from build123d import *

# Parameters (mm, degrees)
SKETCH2_R                        = 21.59
SKETCH2_R_2                      = 10.922
BOSS_EXTRUDE1_DEPTH              = 38.1
CUT_EXTRUDE1_REACH               = 50.825
SKETCH3_W                        = 21.59
SKETCH3_H                        = 1.5875
CUT_EXTRUDE2_REACH               = 50.825
SKETCH4_R                        = 3.0226
TAP_DRILL_FOR_M4X0_7_TAP1_REACH  = 54.717
TAP_DRILL_FOR_M4X0_7_TAP1_BORE_R = 1.65
CUT_EXTRUDE5_REACH               = 63.5
CUT_EXTRUDE5_END_RADIUS          = 3.0226
SKETCH11_R                       = 1.65
CUT_EXTRUDE6_REACH               = 50.825
TAP_DRILL_FOR_M3X0_5_TAP2_D      = 2.5
TAP_DRILL_FOR_M3X0_5_TAP2_DEPTH  = 4.572
TAP_DRILL_FOR_M3X0_5_TAP2_TIP    = 0.751075774


with BuildPart() as part:
    # Sketch2 → Boss-Extrude1 (new body)
    with BuildSketch(Plane(origin=(0, 0, 0), x_dir=(1, 0, 0), z_dir=(0, 1, 0))):
        with Locations(Location((0, 0, 0), (0, 0, 90))):
            Circle(SKETCH2_R)
        with Locations(Location((0, 0, 0), (0, 0, 90))):
            Circle(SKETCH2_R_2, mode=Mode.SUBTRACT)
    extrude(amount=BOSS_EXTRUDE1_DEPTH)

    # Sketch3 → Cut-Extrude1 (cut, up to next)
    with BuildSketch(Plane(origin=(0, 38.1, 0), x_dir=(1, 0, 0), z_dir=(0, 1, 0)), mode=Mode.PRIVATE) as cut_extrude1_sk1:
        with Locations((-10.795, 0)):
            Rectangle(SKETCH3_W, SKETCH3_H)
    cut_extrude1_tool1 = extrude(cut_extrude1_sk1.sketch, amount=-CUT_EXTRUDE1_REACH, mode=Mode.PRIVATE) & part.part
    add(cut_extrude1_tool1.solids().sort_by_distance((-10.795, 38.1, 0))[0], mode=Mode.SUBTRACT)

    # Sketch4 → Cut-Extrude2 (cut, up to next)
    with BuildSketch(Plane(origin=(0, 38.1, 0), x_dir=(1, 0, 0), z_dir=(0, 1, 0)), mode=Mode.PRIVATE) as cut_extrude2_sk1:
        with Locations(Location((0, -16.256, 0), (0, 0, 270))):
            Circle(SKETCH4_R)
    cut_extrude2_tool1 = extrude(cut_extrude2_sk1.sketch, amount=-CUT_EXTRUDE2_REACH, mode=Mode.PRIVATE) & part.part
    cut_extrude2 = cut_extrude2_tool1.solids().sort_by_distance((0, 38.1, 16.256))[0]
    add(cut_extrude2, mode=Mode.SUBTRACT)

    # Tap Drill for M4x0.7 Tap1 bore (on position points) → Tap Drill for M4x0.7 Tap1 (cut, up to next)
    with BuildSketch(Plane(origin=(-16.234261615, 29.109235595, 0.79375), x_dir=(-1, 0, 0), z_dir=(0, 0, -1)), mode=Mode.PRIVATE) as tap_drill_for_m4x0_7_tap1_sk1:
        Circle(TAP_DRILL_FOR_M4X0_7_TAP1_BORE_R)
    tap_drill_for_m4x0_7_tap1_tool1 = extrude(tap_drill_for_m4x0_7_tap1_sk1.sketch, amount=-TAP_DRILL_FOR_M4X0_7_TAP1_REACH, mode=Mode.PRIVATE) & part.part
    # Tap Drill for M4x0.7 Tap1 bore (on position points) → Tap Drill for M4x0.7 Tap1 (cut, up to next)
    with BuildSketch(Plane(origin=(-16.234261615, 29.109235595, 0.79375), x_dir=(-1, 0, 0), z_dir=(0, 0, -1)), mode=Mode.PRIVATE) as tap_drill_for_m4x0_7_tap1_sk2:
        with Locations((0, -20.205281104)):
            Circle(TAP_DRILL_FOR_M4X0_7_TAP1_BORE_R)
    tap_drill_for_m4x0_7_tap1_tool2 = extrude(tap_drill_for_m4x0_7_tap1_sk2.sketch, amount=-TAP_DRILL_FOR_M4X0_7_TAP1_REACH, mode=Mode.PRIVATE) & part.part
    add(tap_drill_for_m4x0_7_tap1_tool1.solids().sort_by_distance((-16.234262, 29.109236, 0.79375))[0], mode=Mode.SUBTRACT)
    add(tap_drill_for_m4x0_7_tap1_tool2.solids().sort_by_distance((-16.234262, 8.903954, 0.79375))[0], mode=Mode.SUBTRACT)

    # Cut-Extrude5: up to this cylinder (the profile starts outside it)
    cut_extrude5_end = Plane(origin=(0, 19.05, 16.256), z_dir=(0, 1, 0)) * Cylinder(CUT_EXTRUDE5_END_RADIUS, 134.0452, mode=Mode.PRIVATE)
    # Sketch11 → Cut-Extrude5 (cut, up to the surface)
    with BuildSketch(Plane.XY.offset(21.59), mode=Mode.PRIVATE) as cut_extrude5_sk1:
        with Locations((0.007297963, 19.05)):
            Circle(SKETCH11_R)
    cut_extrude5_tool1 = extrude(cut_extrude5_sk1.sketch, amount=-CUT_EXTRUDE5_REACH, mode=Mode.PRIVATE) - cut_extrude5_end
    cut_extrude5 = cut_extrude5_tool1.solids().sort_by_distance((0.007298, 19.05, 21.59))[0]
    add(cut_extrude5, mode=Mode.SUBTRACT)

    # Mirror1: Cut-Extrude2, Cut-Extrude5 across plane
    add(cut_extrude2.mirror(Plane.XY), mode=Mode.SUBTRACT)
    add(cut_extrude5.mirror(Plane.XY), mode=Mode.SUBTRACT)

    # Sketch12 → Cut-Extrude6 (cut, up to next)
    with BuildSketch(Plane(origin=(0, 38.1, 0), x_dir=(1, 0, 0), z_dir=(0, 1, 0)), mode=Mode.PRIVATE) as cut_extrude6_sk1:
        with BuildLine():
            Line((20.32, 7.295594561), (20.32, -7.295594561))
            ThreePointArc((20.32, -7.295594561), (21.59, 0), (20.32, 7.295594561))
        make_face()
    cut_extrude6_tool1 = extrude(cut_extrude6_sk1.sketch, amount=-CUT_EXTRUDE6_REACH, mode=Mode.PRIVATE) & part.part
    add(cut_extrude6_tool1.solids().sort_by_distance((20.829303, 38.1, 0))[0], mode=Mode.SUBTRACT)

    # Tap Drill for M3x0.5 Tap2
    with Locations(Plane(origin=(20.32, 19.05, 0), x_dir=(0, 0, 1), z_dir=(1, 0, 0))):
        with Locations((0, 0)):
            Hole(TAP_DRILL_FOR_M3X0_5_TAP2_D / 2, depth=TAP_DRILL_FOR_M3X0_5_TAP2_DEPTH)
            with Locations((0, 0, -(TAP_DRILL_FOR_M3X0_5_TAP2_DEPTH + TAP_DRILL_FOR_M3X0_5_TAP2_TIP / 2))):  # 118° drill point
                Cone(0, TAP_DRILL_FOR_M3X0_5_TAP2_D / 2, TAP_DRILL_FOR_M3X0_5_TAP2_TIP, mode=Mode.SUBTRACT)


solid = part.part
Source: CAD feature listing. Evaluate the final solid. Frame: model axes, mm. A direction names the side the tool comes from. Give positions to 0.01 mm unless a question says otherwise; leave off trailing zeros. Order: outer loops, then holes, each group sorted by start corner. A loop starts at its lowest first (then second) coordinate and runs counter-clockwise, first axis right, second up. Notation, with made-up numbers: (-11.5, 70) -> (19.5, 70) arc R19 cw to (19.5, 87) -> close; hole circle Ø10 at (56, 49.25). An arc over 180 degrees is marked (long way). Write item = value, one per line.
Item 1: Set-up query: faces 4 (the face through (-16, 19, 0.794)), 5 (the face through (0.769, 17.586, 20.207)), 6 (the face through (0.769, 17.586, -20.207)). Return all of +Z, -Z, +X, -X, +Y, -Y with unobstructed straight access to the full face (end or side cutting, diameter ignored); none if empty.
Check result:
face_4 = -X, +Y, -Y
face_5 = +Z
face_6 = -Z
Item 2: Section query C-C (x = -13). Output: boundary loops of the cut face in (y, z).
Check result:
outline = (0, -17.24) -> (38.1, -17.24) -> (38.1, -0.79) -> (0, -0.79) -> close; (0, 0.79) -> (38.1, 0.79) -> (38.1, 17.24) -> (0, 17.24) -> close
Item 3: Section query D-D (z = -12). Output: boundary loops of the cut face in (x, y), then the cut area to 3 significant figures.
Check result:
outline = (-17.95, 0) -> (17.95, 0) -> (17.95, 38.1) -> (-17.95, 38.1) -> close
area = 1,370 mm²
Item 4: Contact query for flat-ended pins moving along their axis: pin 1 (1.5 mm diameter, centred on y = 19.05, z = 0, fed in from +X); pin 2 (4.5 mm diameter, centred on x = -16.23, y = 29.11, fed in from +Z); pin 3 (3 mm diameter, centred on x = -15, y = 22, fed in from -Z); pin 4 (4.5 mm diameter, centred on x = 0.01, y = 19.05, fed in from +Z). Output: stop coordinate, or through.
Check result:
pin_1 = 15.45
pin_2 = 16.45
pin_3 = -16.85
pin_4 = 21.59
Item 5: Section query A-A (y = 24). Output: boundary loops of the cut face in (x, z), then the cut area to 3 significant figures.
Check result:
outline = (-21.58, -0.79) arc R21.59 ccw to (20.32, -7.3) -> (20.32, 7.3) arc R21.59 ccw to (-21.58, 0.79) -> (-10.89, 0.79) arc R10.92 cw (long way) to (-10.89, -0.79) -> close; hole circle Ø6.05 at (0, -16.26); hole circle Ø6.05 at (0, 16.26)
area = 1,000 mm²
Item 6: Mould query, pull axis Z, two halves, no side actions, for faces 1 (the face through (18.002, 17.996, -0.672)), 2 (the face through (-3.723, 18.783, 21.267)), 3 (the face through (-14.586, 29.182, 8.251)). Classes: +Z half, -Z half, draft (parallel to the pull), parting line (faces both ways), or undercut.
Check result:
face_1 = undercut
face_2 = +Z half
face_3 = draft
Item 7: Ray query, probe 1 along Y at (x, z) = (19, 0); probe 2 along Z at (x, y) = (1, 14); probe 3 along Z at (x, y) = (-1.5, 34). Return the intervals inside material, ascending.
Check result:
probe_1 = 0 to 17.8, 20.3 to 38.1
probe_2 = -21.57 to -19.11, -13.4 to -10.88, 10.88 to 13.4, 19.11 to 21.57
probe_3 = -21.54 to -18.88, -13.63 to -10.82, 10.82 to 13.63, 18.88 to 21.54
Item 8: Section query B-B (z = -6.5). Output: boundary loops of the cut face in (x, y).
Check result:
outline = (-20.59, 0) -> (-8.78, 0) -> (-8.78, 38.1) -> (-20.59, 38.1) -> close; (8.78, 0) -> (20.32, 0) -> (20.32, 38.1) -> (8.78, 38.1) -> close
